Can you work these out from the drawing? Everything is in mm from the part's minimum corner. A direction names the side the tool comes from. Give positions to 0.01 mm unless a question says otherwise; leave off trailing zeros. Loops run counter-clockwise (first coordinate to the right, second up) from the corner with the lowest first, then second, coordinate; pieces in that order, holes last. Notation, with made-up numbers: (42.5, -10) -> (66.5, -10) arc R6 cw to (66.5, -4) -> close; hole circle Ø4 at (82, 19.25). An arc over 180 degrees is marked (long way). Write item = value, one per line. Start each with the question number.
1) If we mould it in two halves opening along Z, with no side actions, what happens to the marked faces 1, 2, 3 and 4? For each: +Z half, -Z half, draft (parallel to the pull), parting line (faces both ways), or undercut.
2) I want a section at B-B (z = 2). List the corners of the cut face in (x, y) for me, and give its area (3 significant figures).
3) I need wall thicknesses on probe 1 along Z at (x, y) = (10.75, 41); probe 2 along X at (y, z) = (97, 13.6) (3 decimals). Which ranges of each line are inside material? Lowest first, please. Write a range as from..to.
4) On a 3-axis mill with a long thin cutter (end or side, diameter ignored), from which of +Z, -Z, +X, -X, +Y, -Y can I reach the whole of each face in a straight line? I mean the marked faces 5 and 6. Say none if no direction works.
5) I want a section at A-A (x = 12). List the corners of the cut face in (y, z) for me.
6) I'm going to push flat-ended pins straight in: pin 1 Ø2.5 at (x, y) = (6.925, 3) entering from +Z; pin 2 Ø6 at (y, z) = (48.5, 4.5) entering from -X. Where does each tip first touch, or does it pass through?
7) I want a section at C-C (y = 85). List the corners of the cut face in (x, z) for me (3 decimals), and give its area (3 significant figures).
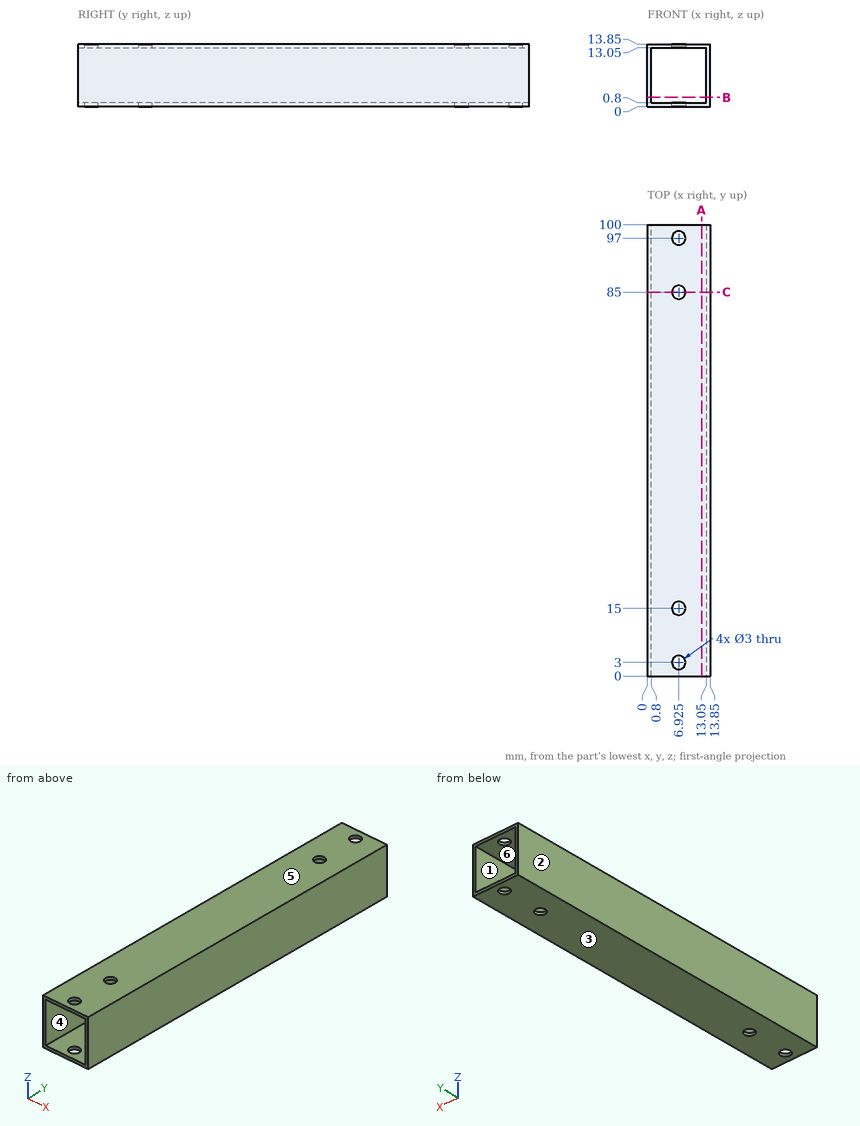
Answer list:
q1.face_1 = undercut
q1.face_2 = draft
q1.face_3 = -Z half
q1.face_4 = undercut
q2.outline = (0, 0) -> (0.8, 0) -> (0.8, 100) -> (0, 100) -> close; (13.05, 0) -> (13.85, 0) -> (13.85, 100) -> (13.05, 100) -> close
q2.area = 160 mm^2
q3.probe_1 = 0..0.8, 13.05..13.85
q3.probe_2 = 0..5.425, 8.425..13.85
q4.face_5 = +Z, +X, -X, +Y, -Y
q4.face_6 = +Y, -Y
q5.outline = (0, 0) -> (100, 0) -> (100, 0.8) -> (0, 0.8) -> close; (0, 13.05) -> (100, 13.05) -> (100, 13.85) -> (0, 13.85) -> close
q6.pin_1 = through
q6.pin_2 = 0
q7.outline = (0, 0) -> (5.425, 0) -> (5.425, 0.8) -> (0.8, 0.8) -> (0.8, 13.05) -> (5.425, 13.05) -> (5.425, 13.85) -> (0, 13.85) -> close; (8.425, 0) -> (13.85, 0) -> (13.85, 13.85) -> (8.425, 13.85) -> (8.425, 13.05) -> (13.05, 13.05) -> (13.05, 0.8) -> (8.425, 0.8) -> close
q7.area = 37.0 mm^2
